from build123d import *

# Parameters (mm, degrees)
F0_W     = 50
F0_H     = 25
F1_DEPTH = 3
F3_D     = 3.2
F4_W     = 31
F4_H     = 22
F5_DEPTH = 0.7
F7_D     = 1.8
F9_DEPTH = 8


with BuildPart() as f1:
    # F0 (on Top) → F1 (new body)
    with BuildSketch(Plane.XY):
        with Locations((25, 11.048387)):
            Rectangle(F0_W, F0_H)
    extrude(amount=F1_DEPTH)

    # F3 (through all)
    with Locations(Plane.XY.offset(3)):
        with Locations((2.12132, 21.427067), (47.87868, 21.427067), (47.87868, 0.669707), (2.12132, 0.669707)):
            Hole(F3_D / 2)

    # F4 (on face) → F5 (cut)
    with BuildSketch(Plane.XY.offset(3)):
        with Locations((25, 11.048387)):
            Rectangle(F4_W, F4_H)
    extrude(amount=-F5_DEPTH, mode=Mode.SUBTRACT)

    # F7 (through all)
    with Locations(Plane.XY.offset(2.3)):
        with Locations((16.5, 3.048387), (35.5, 19.048387)):
            Hole(F7_D / 2)

    # F8 (on face) → F9 (join)
    with BuildSketch(Plane.XY.offset(3)):
        Polygon((49, 15.348387), (49, 14.348387), (50, 14.348387), (50, 16.348387), (49, 16.348387), (45.595244, 16.348387), (45.595244, 15.348387), (45.595244, 6.748387), (45.595244, 5.748387), (49, 5.748387), (50, 5.748387), (50, 7.748387), (49, 7.748387), (49, 6.748387), (46.7, 6.748387), (46.7, 15.348387), align=None)
    extrude(amount=F9_DEPTH)


solid = f1.part
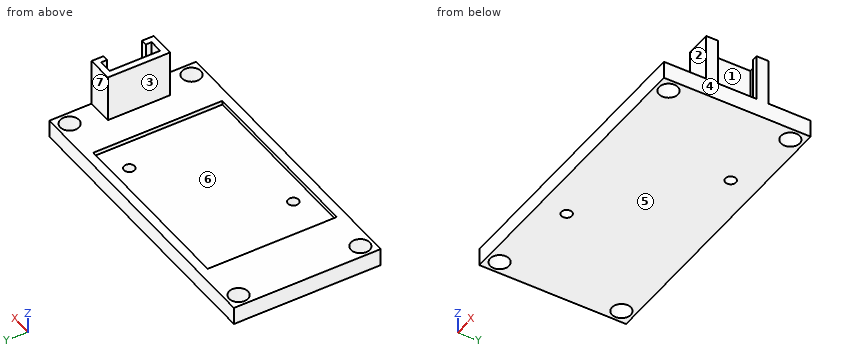
Model file for the job. Use its own axes, mm. Face numbers are marked on the shaded views. A direction names the side the tool comes from. Round coordinates to 2 decimals unless told otherwise and drop trailing zeros. Order: outer loops, then holes, each group sorted by start corner. A loop starts at its lowest first (then second) coordinate and runs counter-clockwise, first axis right, second up.
(1) 3-axis set-ups, long thin cutter, end or side, ignore diameter. For the marked faces 5, 6 and 7: which of +Z, -Z, +X, -X, +Y, -Y reach the whole face in a straight line?
(2) Band-saw the part on D-D (x = 43.5). List the corners of the cut face in (y, z).
(3) Pull direction X, two halves, no side cores. Call the marked faces 1, 2, 3 and 4: released by +X, released by -X, zero draft, split by the parting line, or undercut.
(4) Band-saw the part on A-A (x = 16.5). List the corners of the cut face in (y, z), then the cut area to 3 significant figures.
(5) Band-saw the part on C-C (y = 17.5). List the corners of the cut face in (x, z).
(6) Band-saw the part on B-B (z = 5). List the corners of the cut face in (x, y).
(7) Drill centre lines: line 1 (Y direction, x = 46.5, z = 2.5); line 2 (X direction, y = 1.25, z = 2.5); line 3 (Z direction, x = 25, y = 18.25). Where is each one in solid material? Low to high.
(8) Pin check, flat tips, straight feed: pin 1 (3 mm diameter, centred on x = 15, y = 7.5, fed in from +Z); pin 2 (1.3 mm diameter, centred on x = 48, z = 9, fed in from +Y); pin 3 (1.1 mm diameter, centred on y = 7, z = 7, fed in from -X). Stop position of each tip, or through.
Verdict:
1. face 5: -Z, +X, -X, +Y, -Y
1. face 6: +Z
1. face 7: +Z, +X, -X, +Y
2. outline: (-1.45, 0) - (23.55, 0) - (23.55, 3) - (-1.45, 3) - close
3. face 1: undercut
3. face 2: zero draft
3. face 3: released by -X
3. face 4: released by +X
4. outline: (-1.45, 0) - (2.15, 0) - (2.15, 2.3) - (0.05, 2.3) - (0.05, 3) - (-1.45, 3) - close; (3.95, 0) - (23.55, 0) - (23.55, 3) - (22.05, 3) - (22.05, 2.3) - (3.95, 2.3) - close
4. area: 55.5 mm2
5. outline: (0, 0) - (50, 0) - (50, 3) - (40.5, 3) - (40.5, 2.3) - (9.5, 2.3) - (9.5, 3) - (0, 3) - close
6. outline: (45.6, 5.75) - (50, 5.75) - (50, 7.75) - (49, 7.75) - (49, 6.75) - (46.7, 6.75) - (46.7, 15.35) - (49, 15.35) - (49, 14.35) - (50, 14.35) - (50, 16.35) - (45.6, 16.35) - close
7. line 1: y = -1.45 to -0.14, 1.48 to 20.62, 22.24 to 23.55
7. line 2: x = 0 to 0.63, 3.61 to 9.5, 40.5 to 46.39, 49.37 to 50
7. line 3: z = 0 to 2.3
8. pin 1: stops at z = 2.3
8. pin 2: stops at y = 16.35
8. pin 3: stops at x = 45.6
